```python
from build123d import *

# Parameters (mm, degrees)
SKETCH024_W     = 65.8
SKETCH024_H     = 99.8
PAD016_DEPTH    = 2
SKETCH166_W     = 23.8
SKETCH166_H     = 23.8
SKETCH166_H_2   = 11.8
PAD112_DEPTH    = 3.5
SKETCH302_R     = 0.75
POCKET047_DEPTH = 4


with BuildPart() as part:
    # Sketch024 → Pad016 (new body)
    with BuildSketch(Plane.XZ):
        Rectangle(SKETCH024_W, SKETCH024_H)
        Polygon((8, 38), (-8, 38), (-11, 35), (-8, 32), (8, 32), (11, 35), align=None, mode=Mode.SUBTRACT)
        Polygon((-14.5, 25.5), (-17.5, 28.5), (-20.5, 25.5), (-20.5, 9.5), (-17.5, 6.5), (-14.5, 9.5), align=None, mode=Mode.SUBTRACT)
        Polygon((-14.5, -9.5), (-17.5, -6.5), (-20.5, -9.5), (-20.5, -25.5), (-17.5, -28.5), (-14.5, -25.5), align=None, mode=Mode.SUBTRACT)
        Polygon((8, -32), (-8, -32), (-11, -35), (-8, -38), (8, -38), (11, -35), align=None, mode=Mode.SUBTRACT)
        Polygon((20.5, 25.5), (17.5, 28.5), (14.5, 25.5), (14.5, 9.5), (17.5, 6.5), (20.5, 9.5), align=None, mode=Mode.SUBTRACT)
        Polygon((20.5, -9.5), (17.5, -6.5), (14.5, -9.5), (14.5, -25.5), (17.5, -28.5), (20.5, -25.5), align=None, mode=Mode.SUBTRACT)
        Polygon((8, 3), (-8, 3), (-11, 0), (-8, -3), (8, -3), (11, 0), align=None, mode=Mode.SUBTRACT)
    extrude(amount=PAD016_DEPTH)

    # Sketch166 (on Face48 of Pad016) → Pad112 (join)
    with BuildSketch(Plane.XZ.offset(2)):
        with Locations((0, 17.5)):
            Rectangle(SKETCH166_W, SKETCH166_H)
        with Locations((0, -24)):
            Rectangle(SKETCH166_W, SKETCH166_H_2)
    extrude(amount=PAD112_DEPTH)

    # Sketch302 (on Face58 of Pad112) → Pocket047 (cut)
    with BuildSketch(Plane.XZ.offset(5.5)):
        with Locations((-10, 27.5)):
            Circle(SKETCH302_R)
        with Locations((10, 7.5)):
            Circle(SKETCH302_R)
        with Locations((-10, -20)):
            Circle(SKETCH302_R)
        with Locations((10, -28)):
            Circle(SKETCH302_R)
    extrude(amount=-POCKET047_DEPTH, mode=Mode.SUBTRACT)


with BuildPart() as part_1:
    # Body009 placement: moved
    add(part.part.moved(Location((0, 12, 0))))


solid = part_1.part
```
The listing builds one solid part. Answer for the finished solid, in the listing's coordinates (mm). A direction names the side the tool comes from. Give positions to 0.01 mm unless a question says otherwise; leave off trailing zeros. Order: outer loops, then holes, each group sorted by start corner. A loop starts at its lowest first (then second) coordinate and runs counter-clockwise, first axis right, second up. Notation, with made-up numbers: (18.25, 49.25) - (43.25, 49.25) arc R14 ccw to (43.25, 75.25) - close; hole circle Ø3 at (-2, -14.75). An arc over 180 degrees is marked (long way). Answer in a Markdown table with one row per item. Add a question column.
Q1. The part is cut by section B-B (z = 36). Determine the outline of the cut face in (x, y), then the cut area to 3 significant figures.
Q2. The part is cut by section D-D (x = -25.5). Determine the outline of the cut face in (y, z), then the cut area to 3 significant figures.
Q3. Given P1, Ø1.8, axis at y = 8, z = 13.5, coming from the +X side; P2, Ø3, axis at x = 3, y = 7.5, coming from the +Z side; P3, Ø1, axis at y = 8, z = -26.5, coming from the -X side, each flat-ended and moving along its own axis, determine where each tip first touches the part or whether it passes through.
Q4. Which of the six approach directions +Z, -Z, +X, -X, +Y, -Y give full straight-line access (tool end or side, diameter ignored) to faces 5 (the flat face through (-11.9, 8, 17)), 6 (the flat face through (0, 6.5, -24)), 7 (the flat face through (10, 11, 36))?
Q5. For a pull along Z with two mould halves and no side action, classify faces 1 (the flat face through (19, 11, -27)), 2 (the flat face through (16, 11, -27)), 3 (the flat face through (11.9, 8, 17)), 4 (the flat face through (0, 11, 49.9)) as released by +Z, released by -Z, zero draft, split by the parting line, or undercut.
Q6. Find the intervals of material crossed by line 1 along Z through (x, y) = (-10, 8.15); line 2 along Z through (x, y) = (10, 7.6); line 3 along Y through (x, z) = (-14, 42.5), in increasing order. Write a range as [from, to].
Q7. The part is cut by section A-A (y = 8.1). Determine the outline of the cut face in (x, z), then the cut area to 3 significant figures.
Q8. The part is cut by section C-C (x = 4.5). Determine the outline of the cut face in (y, z).
Determined:
| question | item | result |
|---|---|---|
| 1 | outline | (-32.9, 10) - (-10, 10) - (-10, 12) - (-32.9, 12) - close; (10, 10) - (32.9, 10) - (32.9, 12) - (10, 12) - close |
| 1 | area | 91.6 mm² |
| 2 | outline | (10, -49.9) - (12, -49.9) - (12, 49.9) - (10, 49.9) - close |
| 2 | area | 200 mm² |
| 3 | P1 | stops at x = 11.9 |
| 3 | P2 | stops at z = 29.4 |
| 3 | P3 | stops at x = -11.9 |
| 4 | face 5 | +Z, -Z, -X, -Y |
| 4 | face 6 | +Z, -Z, +X, -X, -Y |
| 4 | face 7 | +Y, -Y |
| 5 | face 1 | undercut |
| 5 | face 2 | undercut |
| 5 | face 3 | zero draft |
| 5 | face 4 | released by +Z |
| 6 | line 1 | z = [-29.9, -20.75], [-19.25, -18.1], [5.6, 26.75], [28.25, 29.4] |
| 6 | line 2 | z = [-29.9, -28.75], [-27.25, -18.1], [5.6, 6.75], [8.25, 29.4] |
| 6 | line 3 | y = [10, 12] |
| 7 | outline | (-11.9, -29.9) - (11.9, -29.9) - (11.9, -18.1) - (-11.9, -18.1) - close; (-11.9, 5.6) - (11.9, 5.6) - (11.9, 29.4) - (-11.9, 29.4) - close; hole circle Ø1.5 at (-10, -20); hole circle Ø1.5 at (-10, 27.5); hole circle Ø1.5 at (10, -28); hole circle Ø1.5 at (10, 7.5) |
| 7 | area | 840 mm² |
| 8 | outline | (6.5, -29.9) - (10, -29.9) - (10, -32) - (12, -32) - (12, -3) - (10, -3) - (10, -18.1) - (6.5, -18.1) - close; (6.5, 5.6) - (10, 5.6) - (10, 3) - (12, 3) - (12, 32) - (10, 32) - (10, 29.4) - (6.5, 29.4) - close; (10, -49.9) - (12, -49.9) - (12, -38) - (10, -38) - close; (10, 38) - (12, 38) - (12, 49.9) - (10, 49.9) - close |
